```python
from build123d import *

# Parameters (mm, degrees)
F0_W      = 33.27
F0_H      = 17.76
F1_DEPTH  = 1.5
F2_W      = 9
F2_H      = 4
F3_DEPTH  = 2
F3_FACE_W = 9
F3_FACE_H = 4
F4_DEPTH  = 7


with BuildPart() as f1:
    # F0 (on Top) → F1 (new body)
    with BuildSketch(Plane.XY):
        Rectangle(F0_W, F0_H)
    extrude(amount=F1_DEPTH)



with BuildPart() as f3:
    # F2 (on face) → F3 (new body)
    with BuildSketch(Plane(origin=(-16.635, 0, 0), x_dir=(0, -1, 0), z_dir=(-1, 0, 0))):
        with Locations((0, 3.5)):
            Rectangle(F2_W, F2_H)
    extrude(amount=F3_DEPTH)


with BuildPart() as f1_1:
    add(f1.part)

    add(f3.part)  # F4 merges F3
    # F3_face (on face) → F4 (join)
    with BuildSketch(Plane(origin=(-16.635, 0, 3.5), x_dir=(0, -1, 0), z_dir=(1, 0, 0))):
        Rectangle(F3_FACE_W, F3_FACE_H)
    extrude(amount=F4_DEPTH)


solid = f1_1.part
```
Model file for the job. Use its own axes, mm. A direction names the side the tool comes from. Round coordinates to 2 decimals unless told otherwise and drop trailing zeros. Order: outer loops, then holes, each group sorted by start corner. A loop starts at its lowest first (then second) coordinate and runs counter-clockwise, first axis right, second up. Notation, with made-up numbers: M 37.5,-14.75 L 96.5,-14.75 A12 cw 96.5,7.25 Z; hole C 12.25,2.25 d6. An arc over 180 degrees is marked long. Use CSV: the item, a comma, the result in double quotes.
Item 1: Saw through at C-C (z = 4.9). List the corners of the cut face in (x, y) (3 decimals), plus the area to 3 significant figures.
Worked answers:
outline,"M -18.635,-4.5 L -9.635,-4.5 L -9.635,4.5 L -18.635,4.5 Z"
area,"81.0 mm²"
Item 2: Which spindle directions (+Z, -Z, +X, -X, +Y, -Y) get a long thin tool onto all of the face, cutting with end or side? Do faces 1 (the face through (-14, 4.5, 4)), 2 (the face through (-14, -4.5, 4)), 3 (the face through (-18, 0, 1.5)). Say none if no direction does.
Worked answers:
face 1,"+Z, +X, -X, +Y"
face 2,"+Z, +X, -X, -Y"
face 3,"-Z, -X, +Y, -Y"
Item 3: Pin check, flat tips, straight feed: pin 1 (0.8 mm diameter, centred on y = 1, z = 1, fed in from -X) (3 decimals); pin 2 (1.2 mm diameter, centred on x = -16, z = 4, fed in from -Y); pin 3 (1 mm diameter, centred on x = -18, y = -2, fed in from -Z). Stop position of each tip, or through.
Worked answers:
pin 1,"x = -16.635"
pin 2,"y = -4.5"
pin 3,"z = 1.5"
Item 4: Saw through at B-B (y = 3.5). List the corners of the cut face in (x, z) (3 decimals).
Worked answers:
outline,"M -18.635,1.5 L -16.635,1.5 L -16.635,0 L 16.635,0 L 16.635,1.5 L -9.635,1.5 L -9.635,5.5 L -18.635,5.5 Z"
Item 5: Saw through at A-A (x = -14). List the corners of the cut face in (y, z), plus the area to 3 significant figures.
Worked answers:
outline,"M -8.88,0 L 8.88,0 L 8.88,1.5 L 4.5,1.5 L 4.5,5.5 L -4.5,5.5 L -4.5,1.5 L -8.88,1.5 Z"
area,"62.6 mm²"
Item 6: Saw through at D-D (y = 5.75). List the corners of the cut face in (x, z) (3 decimals), plus the area to 3 significant figures.
Worked answers:
outline,"M -16.635,0 L 16.635,0 L 16.635,1.5 L -16.635,1.5 Z"
area,"49.9 mm²"
Item 7: Probe probe 1 along Y at (x, z) = (-10.5, 3.7); probe 2 along X at (y, z) = (-4.25, 4.35) (3 decimals); probe 3 along Z at (x, y) = (-8, 0.75). List the from-to ranges inside material, lowest first.
Worked answers:
probe 1,"-4.5 to 4.5"
probe 2,"-18.635 to -9.635"
probe 3,"0 to 1.5"
